from build123d import *

# Parameters (mm, degrees)
SKETCH_1_W          = 140
SKETCH_1_H          = 65
EXTRUDE_1_DEPTH     = 2
SKETCH_2_R          = 1.6
CUT_EXTRUDE_1_DEPTH = 2
CUT_EXTRUDE_2_DEPTH = 2
FILLET_1_R          = 5


with BuildPart() as part:
    # 草图1 → 凸台-拉伸1 (new body)
    with BuildSketch(Plane.XY):
        Rectangle(SKETCH_1_W, SKETCH_1_H)
    extrude(amount=EXTRUDE_1_DEPTH)

    # 草图2 → 切除-拉伸1 (cut)
    with BuildSketch(Plane.XY.offset(2)):
        with Locations((-65, 29)):
            Circle(SKETCH_2_R)
        with Locations(Location((65, 29, 0), (0, 0, 180))):
            Circle(SKETCH_2_R)
        with Locations((65, -29)):
            Circle(SKETCH_2_R)
        with Locations(Location((-65, -29, 0), (0, 0, 180))):
            Circle(SKETCH_2_R)
    extrude(amount=-CUT_EXTRUDE_1_DEPTH, mode=Mode.SUBTRACT)

    # 草图3 → 切除-拉伸2 (cut)
    with BuildSketch(Plane.XY.offset(2)):
        with BuildLine():
            Line((-51, 24), (-51, -24))
            ThreePointArc((-51, -24), (-56, -29), (-61, -24))
            Line((-61, -24), (-61, 24))
            ThreePointArc((-61, 24), (-56, 29), (-51, 24))
        make_face()
        with BuildLine():
            Line((-37, 24), (-37, -24))
            ThreePointArc((-37, -24), (-42, -29), (-47, -24))
            Line((-47, -24), (-47, 24))
            ThreePointArc((-47, 24), (-42, 29), (-37, 24))
        make_face()
        with BuildLine():
            Line((-23, 24), (-23, -24))
            ThreePointArc((-23, -24), (-28, -29), (-33, -24))
            Line((-33, -24), (-33, 24))
            ThreePointArc((-33, 24), (-28, 29), (-23, 24))
        make_face()
        with BuildLine():
            Line((-9, 24), (-9, -24))
            ThreePointArc((-9, -24), (-14, -29), (-19, -24))
            Line((-19, -24), (-19, 24))
            ThreePointArc((-19, 24), (-14, 29), (-9, 24))
        make_face()
        with BuildLine():
            Line((5, 24), (5, -24))
            ThreePointArc((5, -24), (0, -29), (-5, -24))
            Line((-5, -24), (-5, 24))
            ThreePointArc((-5, 24), (0, 29), (5, 24))
        make_face()
        with BuildLine():
            Line((19, 24), (19, -24))
            ThreePointArc((19, -24), (14, -29), (9, -24))
            Line((9, -24), (9, 24))
            ThreePointArc((9, 24), (14, 29), (19, 24))
        make_face()
        with BuildLine():
            Line((33, 24), (33, -24))
            ThreePointArc((33, -24), (28, -29), (23, -24))
            Line((23, -24), (23, 24))
            ThreePointArc((23, 24), (28, 29), (33, 24))
        make_face()
        with BuildLine():
            Line((47, 24), (47, -24))
            ThreePointArc((47, -24), (42, -29), (37, -24))
            Line((37, -24), (37, 24))
            ThreePointArc((37, 24), (42, 29), (47, 24))
        make_face()
        with BuildLine():
            Line((61, 24), (61, -24))
            ThreePointArc((61, -24), (56, -29), (51, -24))
            Line((51, -24), (51, 24))
            ThreePointArc((51, 24), (56, 29), (61, 24))
        make_face()
    extrude(amount=-CUT_EXTRUDE_2_DEPTH, mode=Mode.SUBTRACT)

    # 圆角1
    fillet_1_edges = [part.edges().sort_by_distance(p)[0] for p in [
        (-70, 32.5, 1),
        (70, 32.5, 1),
        (70, -32.5, 1),
        (-70, -32.5, 1),
    ]]
    fillet(fillet_1_edges, radius=FILLET_1_R)


solid = part.part
Build history of the part. All positions in model axes, mm. A direction names the side the tool comes from. Give positions to 0.01 mm unless a question says otherwise; leave off trailing zeros. Loops run counter-clockwise (first coordinate to the right, second up) from the corner with the lowest first, then second, coordinate; pieces in that order, holes last. Notation, with made-up numbers: (71.25, 24.25) - (130.25, 24.25) arc R28 ccw to (130.25, 44.25) - close; hole circle Ø3 at (58.25, 49.5). An arc over 180 degrees is marked (long way). Write item = value, one per line. Start each with the question number.
1) Band-saw the part on D-D on x = -14. Give the cut face in (y, z), plus the area to 3 significant figures.
2) Probe probe 1 along Y at (x, z) = (-65, 1.15); probe 2 along Y at (x, z) = (-55.5, 0.9); probe 3 along Y at (x, z) = (64.5, 1.5). List the from-to ranges inside material, lowest first. Write a range as from..to.
3) Pull direction X, two halves, no side cores. Call faces 1 (the flat face through (-17, 29, 2)), 2 (the cylindrical face through (-68.57, -31, 1.01)), 3 (the cylindrical face through (-28, 29, 1)): +X half, -X half, draft (parallel to the pull), parting line (faces both ways), or undercut.
4) Tool access for faces 4 (the cylindrical face through (-68.57, 31, 1.01)), 5 (the cylindrical face through (28, -29, 1)): list every direction of +Z, -Z, +X, -X, +Y, -Y with a clear straight run to the whole face (end or side of a thin tool).
5) Band-saw the part on A-A on x = -39. Give the cut face in (y, z), plus the area to 3 significant figures.
6) Band-saw the part on B-B on y = 0. Count the separate pieces of the cut face and the enclosed holes in it, plus the area to 3 significant figures.
Final values:
q1.outline = (-32.5, 0) - (-29, 0) - (-29, 2) - (-32.5, 2) - close; (29, 0) - (32.5, 0) - (32.5, 2) - (29, 2) - close
q1.area = 14.0 mm²
q2.probe_1 = -32.5..-30.6, -27.4..27.4, 30.6..32.5
q2.probe_2 = -32.5..-28.97, 28.97..32.5
q2.probe_3 = -32.5..-30.52, -27.48..27.48, 30.52..32.5
q3.face_1 = draft
q3.face_2 = -X half
q3.face_3 = undercut
q4.face_4 = +Z, -Z, -X, +Y
q4.face_5 = +Z, -Z
q5.outline = (-32.5, 0) - (-28, 0) - (-28, 2) - (-32.5, 2) - close; (28, 0) - (32.5, 0) - (32.5, 2) - (28, 2) - close
q5.area = 18.0 mm²
q6.separate_pieces = 10
q6.enclosed_holes = 0
q6.area = 100 mm²
